The drawing under review shows one solid part. Ordinate dimensions are in mm from its lowest x, y, z. Coordinates: 2 decimals unless noted, no trailing zeros. Write each loop counter-clockwise with the first axis right and the second up, starting at its lowest first coordinate (ties: lowest second). Pieces come first, ordered by that corner, then holes. Notation, with made-up numbers: (-25.5, 9) - (-14.5, 9) arc R26 cw to (-14.5, 24) - close; hole circle Ø4 at (88.5, 2). An arc over 180 degrees is marked (long way). Use a Markdown table: item, result.
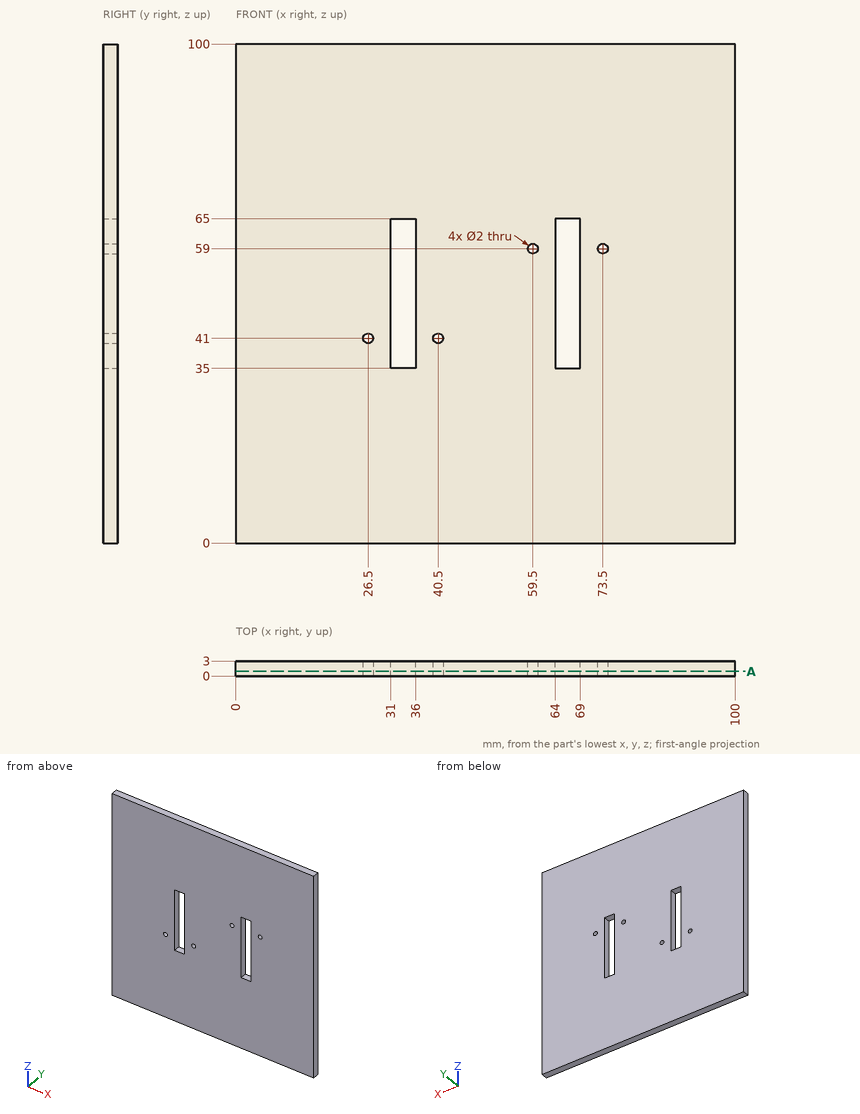
(1) For L1, parallel to X at y = 1.25, z = 41; L2, parallel to X at y = 2.8, z = 38; L3, parallel to Z at x = 40.5, y = 1.3, list the stretches that pass through material, from the lowest coordinate up. Write a range as from..to.
Determined:
| item | result |
|---|---|
| L1 | 0..25.5, 27.5..31, 36..39.5, 41.5..64, 69..100 |
| L2 | 0..31, 36..64, 69..100 |
| L3 | 0..40, 42..100 |
(2) Take a section at A-A on y = 0.95. Write out the cut boundary in (x, z).
Determined:
| item | result |
|---|---|
| outline | (0, 0) - (100, 0) - (100, 100) - (0, 100) - close; hole circle Ø2 at (26.5, 41); hole (31, 35) - (36, 35) - (36, 65) - (31, 65) - close; hole circle Ø2 at (40.5, 41); hole circle Ø2 at (59.5, 59); hole (64, 35) - (69, 35) - (69, 65) - (64, 65) - close; hole circle Ø2 at (73.5, 59) |
(3) For pin 1 (1.2 mm diameter, centred on x = 26.5, z = 41, fed in from +Y); pin 2 (1.5 mm diameter, centred on x = 66.5, y = 2, fed in from -Z), all flat-tipped, find the tip position at first contact; note any pin that passes through.
Determined:
| item | result |
|---|---|
| pin 1 | through |
| pin 2 | z = 0 |
